Verification items for this drawing (mm, ordinates from the low corner). A direction names the side the tool comes from. Coordinates: 2 decimals unless noted, no trailing zeros. Order: outer loops, then holes, each group sorted by start corner. A loop starts at its lowest first (then second) coordinate and runs counter-clockwise, first axis right, second up. Notation, with made-up numbers: (43.25, 83.25) -> (93.25, 83.25) arc R21 cw to (93.25, 108.25) -> close; hole circle Ø3 at (41, -15.75). An arc over 180 degrees is marked (long way). Put each result on its own line as item: value. Start each with the question number.
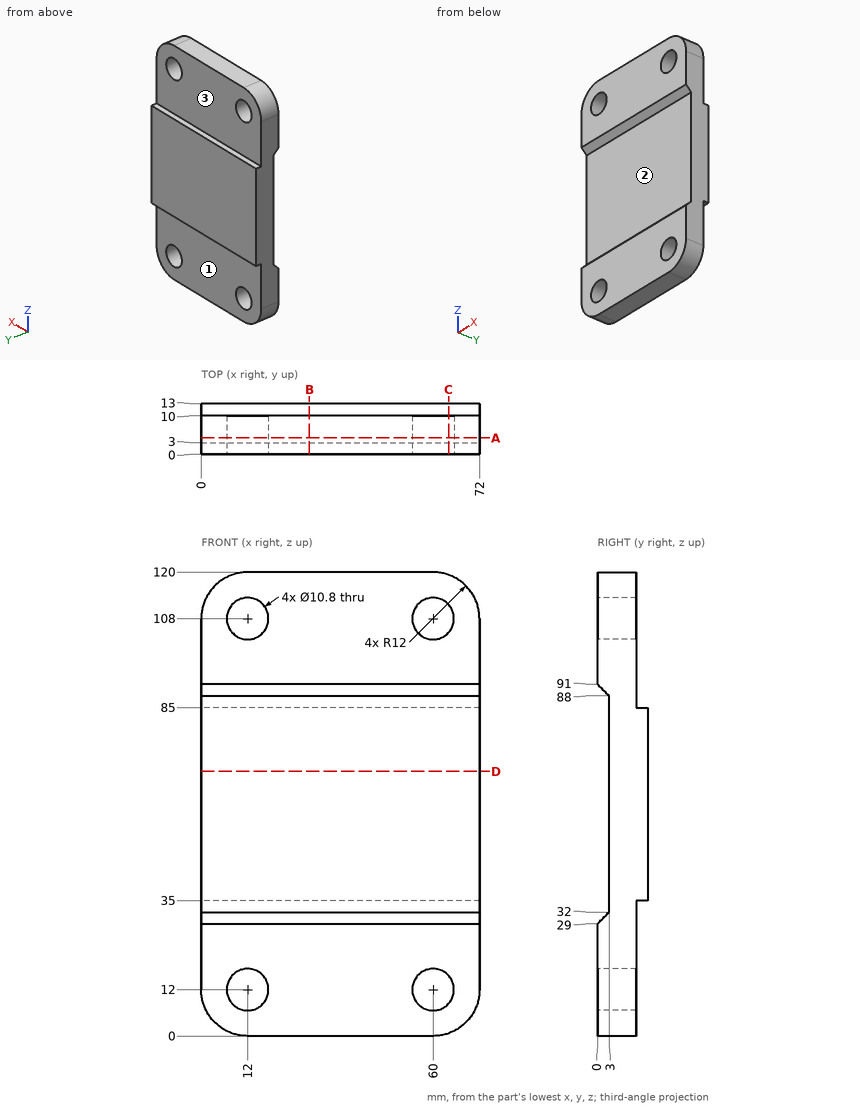
1) Gauge pin test, flat ends, axial feed: pin 1 (14 mm diameter, centred on x = 12, z = 108, fed in from +Y); pin 2 (3.5 mm diameter, centred on x = 18.5, y = 12, fed in from +Z); pin 3 (4 mm diameter, centred on x = 54, z = 67.5, fed in from -Y); pin 4 (6.5 mm diameter, centred on x = 60, z = 108, fed in from +Y). Record the tip position at first contact, or that the pin passes through.
2) Sectioned sample at D-D (z = 68.5). Record the boundary of the cut face in (x, y), plus the area to 3 significant figures.
3) Sectioned sample at C-C (x = 64). Record the boundary of the cut face in (y, z).
4) Scan lines: line 1 along X through (y, z) = (7.75, 12); line 2 along Z through (x, y) = (12, 4.5); line 3 along Z through (x, y) = (12, 2.5). Record each from-to range of solid material in increasing order. Write a range as [from, to].
5) Sectioned sample at A-A (y = 4.25). Record the boundary of the cut face in (x, z).
6) Access from +Z, -Z, +X, -X, +Y, -Y to the whole of each face (thin tool, end or side, straight path). Record for the marked faces 1, 2 and 3.
7) Sectioned sample at B-B (x = 28). Record the boundary of the cut face in (y, z).
Entries:
1. pin 1: stops at y = 10
1. pin 2: stops at z = 85
1. pin 3: stops at y = 3
1. pin 4: passes through
2. outline: (0, 3) -> (72, 3) -> (72, 13) -> (0, 13) -> close
2. area: 720 mm2
3. outline: (0, 0.69) -> (10, 0.69) -> (10, 8.37) -> (0, 8.37) -> close; (0, 15.63) -> (10, 15.63) -> (10, 35) -> (13, 35) -> (13, 85) -> (10, 85) -> (10, 104.37) -> (0, 104.37) -> (0, 91) -> (3, 88) -> (3, 32) -> (0, 29) -> close; (0, 111.63) -> (10, 111.63) -> (10, 119.31) -> (0, 119.31) -> close
4. line 1: x = [0, 6.6], [17.4, 54.6], [65.4, 72]
4. line 2: z = [0, 6.6], [17.4, 102.6], [113.4, 120]
4. line 3: z = [0, 6.6], [17.4, 31.5], [88.5, 102.6], [113.4, 120]
5. outline: (0, 12) arc R12 ccw to (12, 0) -> (60, 0) arc R12 ccw to (72, 12) -> (72, 108) arc R12 ccw to (60, 120) -> (12, 120) arc R12 ccw to (0, 108) -> close; hole circle Ø10.8 at (12, 12); hole circle Ø10.8 at (12, 108); hole circle Ø10.8 at (60, 12); hole circle Ø10.8 at (60, 108)
6. face 1: -Z, +X, -X, +Y
6. face 2: +X, -X, -Y
6. face 3: +Z, +X, -X, +Y
7. outline: (0, 0) -> (10, 0) -> (10, 35) -> (13, 35) -> (13, 85) -> (10, 85) -> (10, 120) -> (0, 120) -> (0, 91) -> (3, 88) -> (3, 32) -> (0, 29) -> close
